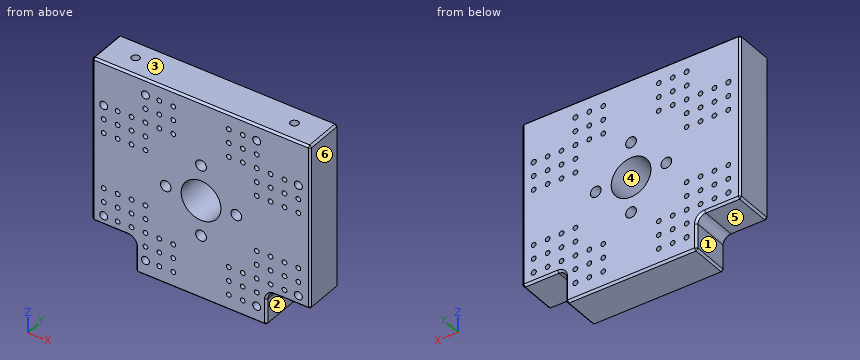
from build123d import *

# Parameters (mm, degrees)
F0_R           = 6
F0_R_2         = 13.5
F0_R_3         = 50
F1_DEPTH       = 100
F3_D           = 13
F3_CBORE_D     = 20
F3_CBORE_DEPTH = 20
F4_SIZE        = 5
F6_D           = 20
F6_DEPTH       = 40
F6_TIP         = 6.0086061903


with BuildPart() as f1:
    # F0 (on Front) → F1 (new body)
    with BuildSketch(Plane.XZ):
        with BuildLine():
            Line((275, 250), (-275, 250))
            Line((-275, 250), (-275, -164))
            Line((-275, -164), (-185, -164))
            ThreePointArc((-185, -164), (-170.8578643763, -169.8578643763), (-165, -184))
            Line((-165, -184), (-165, -250))
            Line((-165, -250), (165, -250))
            Line((165, -250), (165, -184))
            ThreePointArc((165, -184), (170.8578643763, -169.8578643763), (185, -164))
            Line((185, -164), (275, -164))
            Line((275, -164), (275, 250))
        make_face()
        with Locations((-140, -210)):
            Circle(F0_R, mode=Mode.SUBTRACT)
        with Locations((-245, -140)):
            Circle(F0_R, mode=Mode.SUBTRACT)
        with Locations((-210, -140)):
            Circle(F0_R, mode=Mode.SUBTRACT)
        with Locations((-140, -175)):
            Circle(F0_R, mode=Mode.SUBTRACT)
        with Locations((-175, -140)):
            Circle(F0_R, mode=Mode.SUBTRACT)
        with Locations((-140, -140)):
            Circle(F0_R, mode=Mode.SUBTRACT)
        with Locations((-105, -210)):
            Circle(F0_R, mode=Mode.SUBTRACT)
        with Locations((-70, -210)):
            Circle(F0_R, mode=Mode.SUBTRACT)
        with Locations((-105, -175)):
            Circle(F0_R, mode=Mode.SUBTRACT)
        with Locations((-70, -175)):
            Circle(F0_R, mode=Mode.SUBTRACT)
        with Locations((-105, -140)):
            Circle(F0_R, mode=Mode.SUBTRACT)
        with Locations((-70, -140)):
            Circle(F0_R, mode=Mode.SUBTRACT)
        with Locations((-245, -105)):
            Circle(F0_R, mode=Mode.SUBTRACT)
        with Locations((-210, -105)):
            Circle(F0_R, mode=Mode.SUBTRACT)
        with Locations((-245, -70)):
            Circle(F0_R, mode=Mode.SUBTRACT)
        with Locations((-210, -70)):
            Circle(F0_R, mode=Mode.SUBTRACT)
        with Locations((-175, -105)):
            Circle(F0_R, mode=Mode.SUBTRACT)
        with Locations((-140, -105)):
            Circle(F0_R, mode=Mode.SUBTRACT)
        with Locations((-175, -70)):
            Circle(F0_R, mode=Mode.SUBTRACT)
        with Locations((-140, -70)):
            Circle(F0_R, mode=Mode.SUBTRACT)
        with Locations((70, -210)):
            Circle(F0_R, mode=Mode.SUBTRACT)
        with Locations((105, -210)):
            Circle(F0_R, mode=Mode.SUBTRACT)
        with Locations((70, -175)):
            Circle(F0_R, mode=Mode.SUBTRACT)
        with Locations((105, -175)):
            Circle(F0_R, mode=Mode.SUBTRACT)
        with Locations((70, -140)):
            Circle(F0_R, mode=Mode.SUBTRACT)
        with Locations((105, -140)):
            Circle(F0_R, mode=Mode.SUBTRACT)
        with Locations((140, -210)):
            Circle(F0_R, mode=Mode.SUBTRACT)
        with Locations((140, -175)):
            Circle(F0_R, mode=Mode.SUBTRACT)
        with Locations((140, -140)):
            Circle(F0_R, mode=Mode.SUBTRACT)
        with Locations((175, -140)):
            Circle(F0_R, mode=Mode.SUBTRACT)
        with Locations((210, -140)):
            Circle(F0_R, mode=Mode.SUBTRACT)
        with Locations((245, -140)):
            Circle(F0_R, mode=Mode.SUBTRACT)
        with Locations((0, -88.9)):
            Circle(F0_R_2, mode=Mode.SUBTRACT)
        with Locations((140, -105)):
            Circle(F0_R, mode=Mode.SUBTRACT)
        with Locations((175, -105)):
            Circle(F0_R, mode=Mode.SUBTRACT)
        with Locations((140, -70)):
            Circle(F0_R, mode=Mode.SUBTRACT)
        with Locations((175, -70)):
            Circle(F0_R, mode=Mode.SUBTRACT)
        with Locations((210, -105)):
            Circle(F0_R, mode=Mode.SUBTRACT)
        with Locations((245, -105)):
            Circle(F0_R, mode=Mode.SUBTRACT)
        with Locations((210, -70)):
            Circle(F0_R, mode=Mode.SUBTRACT)
        with Locations((245, -70)):
            Circle(F0_R, mode=Mode.SUBTRACT)
        with Locations((-245, 70)):
            Circle(F0_R, mode=Mode.SUBTRACT)
        with Locations((-210, 70)):
            Circle(F0_R, mode=Mode.SUBTRACT)
        with Locations((-245, 105)):
            Circle(F0_R, mode=Mode.SUBTRACT)
        with Locations((-210, 105)):
            Circle(F0_R, mode=Mode.SUBTRACT)
        with Locations((-175, 70)):
            Circle(F0_R, mode=Mode.SUBTRACT)
        with Locations((-140, 70)):
            Circle(F0_R, mode=Mode.SUBTRACT)
        with Locations((-175, 105)):
            Circle(F0_R, mode=Mode.SUBTRACT)
        with Locations((-140, 105)):
            Circle(F0_R, mode=Mode.SUBTRACT)
        with Locations((-88.9, 0)):
            Circle(F0_R_2, mode=Mode.SUBTRACT)
        with Locations((-245, 140)):
            Circle(F0_R, mode=Mode.SUBTRACT)
        with Locations((-210, 140)):
            Circle(F0_R, mode=Mode.SUBTRACT)
        with Locations((-175, 140)):
            Circle(F0_R, mode=Mode.SUBTRACT)
        with Locations((-140, 140)):
            Circle(F0_R, mode=Mode.SUBTRACT)
        with Locations((-140, 175)):
            Circle(F0_R, mode=Mode.SUBTRACT)
        with Locations((-140, 210)):
            Circle(F0_R, mode=Mode.SUBTRACT)
        with Locations((-105, 140)):
            Circle(F0_R, mode=Mode.SUBTRACT)
        with Locations((-70, 140)):
            Circle(F0_R, mode=Mode.SUBTRACT)
        with Locations((-105, 175)):
            Circle(F0_R, mode=Mode.SUBTRACT)
        with Locations((-70, 175)):
            Circle(F0_R, mode=Mode.SUBTRACT)
        with Locations((-105, 210)):
            Circle(F0_R, mode=Mode.SUBTRACT)
        with Locations((-70, 210)):
            Circle(F0_R, mode=Mode.SUBTRACT)
        Circle(F0_R_3, mode=Mode.SUBTRACT)
        with Locations((88.9, 0)):
            Circle(F0_R_2, mode=Mode.SUBTRACT)
        with Locations((0, 88.9)):
            Circle(F0_R_2, mode=Mode.SUBTRACT)
        with Locations((140, 70)):
            Circle(F0_R, mode=Mode.SUBTRACT)
        with Locations((175, 70)):
            Circle(F0_R, mode=Mode.SUBTRACT)
        with Locations((140, 105)):
            Circle(F0_R, mode=Mode.SUBTRACT)
        with Locations((175, 105)):
            Circle(F0_R, mode=Mode.SUBTRACT)
        with Locations((210, 70)):
            Circle(F0_R, mode=Mode.SUBTRACT)
        with Locations((245, 70)):
            Circle(F0_R, mode=Mode.SUBTRACT)
        with Locations((210, 105)):
            Circle(F0_R, mode=Mode.SUBTRACT)
        with Locations((245, 105)):
            Circle(F0_R, mode=Mode.SUBTRACT)
        with Locations((70, 140)):
            Circle(F0_R, mode=Mode.SUBTRACT)
        with Locations((105, 140)):
            Circle(F0_R, mode=Mode.SUBTRACT)
        with Locations((70, 175)):
            Circle(F0_R, mode=Mode.SUBTRACT)
        with Locations((105, 175)):
            Circle(F0_R, mode=Mode.SUBTRACT)
        with Locations((70, 210)):
            Circle(F0_R, mode=Mode.SUBTRACT)
        with Locations((105, 210)):
            Circle(F0_R, mode=Mode.SUBTRACT)
        with Locations((140, 140)):
            Circle(F0_R, mode=Mode.SUBTRACT)
        with Locations((175, 140)):
            Circle(F0_R, mode=Mode.SUBTRACT)
        with Locations((140, 175)):
            Circle(F0_R, mode=Mode.SUBTRACT)
        with Locations((210, 140)):
            Circle(F0_R, mode=Mode.SUBTRACT)
        with Locations((245, 140)):
            Circle(F0_R, mode=Mode.SUBTRACT)
        with Locations((140, 210)):
            Circle(F0_R, mode=Mode.SUBTRACT)
    extrude(amount=F1_DEPTH)

    # F3 (through all)
    with Locations(Plane.XZ.offset(100)):
        with Locations((-245, 140), (245, 140), (245, -140), (-245, -140), (-140, 210), (140, -210), (-140, -210), (140, 210)):
            CounterBoreHole(F3_D / 2, F3_CBORE_D / 2, F3_CBORE_DEPTH)

    # F4
    f4_edges = [f1.edges().sort_by_distance(p)[0] for p in [
        (-275, -100, 43),
        (0, -100, 250),
        (275, -100, 43),
        (230, -100, -164),
        (0, -100, -250),
        (-165, -100, -217),
        (275, 0, 43),
        (0, 0, 250),
        (275, -50, 250),
        (230, 0, -164),
        (0, 0, -250),
        (-170.857864, 0, -169.857864),
        (-275, -50, -164),
        (-275, 0, 43),
        (-165, -50, -250),
        (165, -50, -250),
        (275, -50, -164),
        (-275, -50, 250),
    ]]
    chamfer(f4_edges, length=F4_SIZE)

    # F6
    with Locations(Plane.XY.offset(250)):
        with Locations((-200, -50), (200, -50)):
            Hole(F6_D / 2, depth=F6_DEPTH)
            with Locations((0, 0, -(F6_DEPTH + F6_TIP / 2))):  # 118° drill point
                Cone(0, F6_D / 2, F6_TIP, mode=Mode.SUBTRACT)


solid = f1.part
Verification items for the finished model (mm, model axes). Face numbers are marked on the shaded views. A direction names the side the tool comes from. Coordinates: 2 decimals unless noted, no trailing zeros. Order: outer loops, then holes, each group sorted by start corner. A loop starts at its lowest first (then second) coordinate and runs counter-clockwise, first axis right, second up.
Item 1: Section check B-B, the plane x = 88.9. Enter the section's corners in (y, z).
Filled in:
outline: (-100, -245) - (-95, -250) - (-5, -250) - (0, -245) - (0, -13.5) - (-100, -13.5) - close; (-100, 13.5) - (0, 13.5) - (0, 245) - (-5, 250) - (-95, 250) - (-100, 245) - close
Item 2: Access from +Z, -Z, +X, -X, +Y, -Y to the whole of each face (thin tool, end or side, straight path). Record for the marked faces 1, 2 and 3.
Filled in:
face 1: -Z, -X, +Y, -Y
face 2: -Z, +X, +Y, -Y
face 3: +Z, +X, -X, +Y, -Y
Item 3: Section check D-D, the plane x = -140. Give the number of separate pieces and of enclosed holes in the cut face, then the cut area to 3 significant figures.
Filled in:
separate pieces: 11
enclosed holes: 0
area: 37,500 mm2
Item 4: Section check A-A, the plane z = 0. Enter the section's corners in (x, y), then the cut area to 4 significant figures.
Filled in:
outline: (-275, -95) - (-270, -100) - (-102.4, -100) - (-102.4, 0) - (-270, 0) - (-275, -5) - close; (-75.4, -100) - (-50, -100) - (-50, 0) - (-75.4, 0) - close; (50, -100) - (75.4, -100) - (75.4, 0) - (50, 0) - close; (102.4, -100) - (270, -100) - (275, -95) - (275, -5) - (270, 0) - (102.4, 0) - close
area: 39,550 mm2
Item 5: Section check C-C, the plane z = 88.9. Enter the section's corners in (x, y).
Filled in:
outline: (-275, -95) - (-270, -100) - (-13.5, -100) - (-13.5, 0) - (-270, 0) - (-275, -5) - close; (13.5, -100) - (270, -100) - (275, -95) - (275, -5) - (270, 0) - (13.5, 0) - close
Item 6: Depth check by flat-ended pin: pin 1 (15.5 mm diameter, centred on x = 175, z = -70, fed in from +Y); pin 2 (12 mm diameter, centred on y = -12, z = -188.5, fed in from +X); pin 3 (16 mm diameter, centred on x = -245, z = -140, fed in from -Y). Enter the tip coordinate at first touch or a pass-through.
Filled in:
pin 1: stops at y = 0
pin 2: stops at x = 165.06
pin 3: stops at y = -80
Item 7: Release check for a two-part mould opening along X. For the marked faces 4, 5 and 6 record: +X half, -X half, draft (parallel to the pull), parting line (faces both ways), or undercut.
Filled in:
face 4: undercut
face 5: draft
face 6: +X half
Item 8: Material ranges on L1, parallel to Z at x = 11, y = -14 (3 decimals); L2, parallel to Z at x = 26, y = -75.5; L3, parallel to Z at x = -9, y = -16, recorded low to high.
Filled in:
L1: z = -250 to -96.726, -81.074 to -48.775, 48.775 to 81.074, 96.726 to 250
L2: z = -250 to -42.71, 42.71 to 250
L3: z = -250 to -98.96, -78.84 to -49.18, 49.18 to 78.84, 98.96 to 250
